Work out the finished part from the listing and answer in its coordinate system (mm). A direction names the side the tool comes from. Coordinates: 2 decimals unless noted, no trailing zeros. Order: outer loops, then holes, each group sorted by start corner. A loop starts at its lowest first (then second) coordinate and runs counter-clockwise, first axis right, second up. Notation, with made-up numbers: (32.25, 62) -> (77.25, 62) arc R23 ccw to (77.25, 81) -> close; hole circle Ø6 at (5.5, 32.5). An arc over 180 degrees is marked (long way). Write item = value, one per line. Start each with the question number.
Q1. The part is cut by section B-B, the plane x = -7. Determine the outline of the cut face in (y, z), plus the area to 3 significant figures.
Q2. Flat-ended cylindrical pins translate along their axes: pin 1 (4.5 mm diameter, centred on x = 5, z = -9, fed in from -Y); pin 2 (2.5 mm diameter, centred on x = -5, z = 14, fed in from +Y). Find the tip coordinate at first contact, or state that the pin passes through.
Q3. The part is cut by section D-D, the plane z = 6.5. Determine the outline of the cut face in (x, y).
Q4. The part is cut by section C-C, the plane x = 5. Determine the outline of the cut face in (y, z).
Q5. For a pull along Z with two mould halves and no side action, classify faces 3 (the flat face through (-1, 0, 0)), 4 (the cylindrical face through (-8, 1, 17)), 5 (the cylindrical face through (-8.2, 0.7, -10.6)) as +Z half, -Z half, draft (parallel to the pull), parting line (faces both ways), or undercut.
Q6. The part is cut by section A-A, the plane y = 0.4. Determine the outline of the cut face in (x, z), plus the area to 3 significant figures.
Q7. Straight lines are drawn through the part: L1, parallel to X at y = 1, z = -9; L2, parallel to Z at x = 3.75, y = 0.25; L3, parallel to Z at x = 6, y = 0.25. For each, find the intervals that lie inside material, in ascending order. Write a range as from..to.
Q8. Which of the six approach directions +Z, -Z, +X, -X, +Y, -Y give full straight-line access (tool end or side, diameter ignored) to faces 1 (the flat face through (-9, 1, 9)), 2 (the flat face through (-1, 1.5, 0))?
```python
from build123d import *

# Parameters (mm, degrees)
SKETCH_1_R      = 1.5
SKETCH_1_R_2    = 2
EXTRUDE_1_DEPTH = 1.5
FILLET_1_R      = 5


with BuildPart() as part:
    # ｽｹｯﾁ1 → ﾎﾞｽ - 押し出し1 (new body)
    with BuildSketch(Plane(origin=(0, 0, 0), x_dir=(1, 0, 0), z_dir=(0, 1, 0))):
        with BuildLine():
            Line((-9, -4), (-9, -19))
            Line((-9, -19), (9, -19))
            Line((9, -19), (9, 9))
            ThreePointArc((9, 9), (-1.812547294, 18.966933676), (-10.867953379, 7.380279002))
            Line((-10.867953379, 7.380279002), (-9, -4))
        make_face()
        with Locations(Location((-5, -14, 0), (0, 0, 270))):
            Circle(SKETCH_1_R, mode=Mode.SUBTRACT)
        with Locations(Location((5, -14, 0), (0, 0, 270))):
            Circle(SKETCH_1_R, mode=Mode.SUBTRACT)
        with Locations(Location((-7, 9, 0), (0, 0, 270))):
            Circle(SKETCH_1_R_2, mode=Mode.SUBTRACT)
        with Locations(Location((5, 9, 0), (0, 0, 270))):
            Circle(SKETCH_1_R_2, mode=Mode.SUBTRACT)
    extrude(amount=EXTRUDE_1_DEPTH)

    # ﾌｨﾚｯﾄ1
    fillet_1_edges = [part.edges().sort_by_distance(p)[0] for p in [
        (9, 0.75, 19),
        (-9, 0.75, 19),
        (-9, 0.75, 4),
    ]]
    fillet(fillet_1_edges, radius=FILLET_1_R)


solid = part.part
```
Model answer:
q1.outline = (0, -17) -> (1.5, -17) -> (1.5, -11) -> (0, -11) -> close; (0, -7) -> (1.5, -7) -> (1.5, 18) -> (0, 18) -> close
q1.area = 46.5 mm2
q2.pin_1 = 0
q2.pin_2 = through
q3.outline = (-9, 0) -> (9, 0) -> (9, 1.5) -> (-9, 1.5) -> close
q4.outline = (0, -17) -> (1.5, -17) -> (1.5, -11) -> (0, -11) -> close; (0, -7) -> (1.5, -7) -> (1.5, 12.5) -> (0, 12.5) -> close; (0, 15.5) -> (1.5, 15.5) -> (1.5, 18.9) -> (0, 18.9) -> close
q5.face_3 = draft
q5.face_4 = +Z half
q5.face_5 = undercut
q6.outline = (-10.87, -7.38) arc R10 ccw (long way) to (9, -9) -> (9, 14) arc R5 ccw to (4, 19) -> (-4, 19) arc R5 ccw to (-9, 14) -> (-9, 4.41) arc R5 cw to (-9.07, 3.6) -> close; hole circle Ø4 at (-7, -9); hole circle Ø3 at (-5, 14); hole circle Ø4 at (5, -9); hole circle Ø3 at (5, 14)
q6.area = 625 mm2
q7.L1 = -11..-9, -5..3, 7..9
q7.L2 = -17.8..-10.56, -7.44..13.17, 14.83..19
q7.L3 = -16.14..-10.73, -7.27..12.88, 15.12..18.58
q8.face_1 = +Z, -X, +Y, -Y
q8.face_2 = +Z, -Z, +X, -X, +Y
